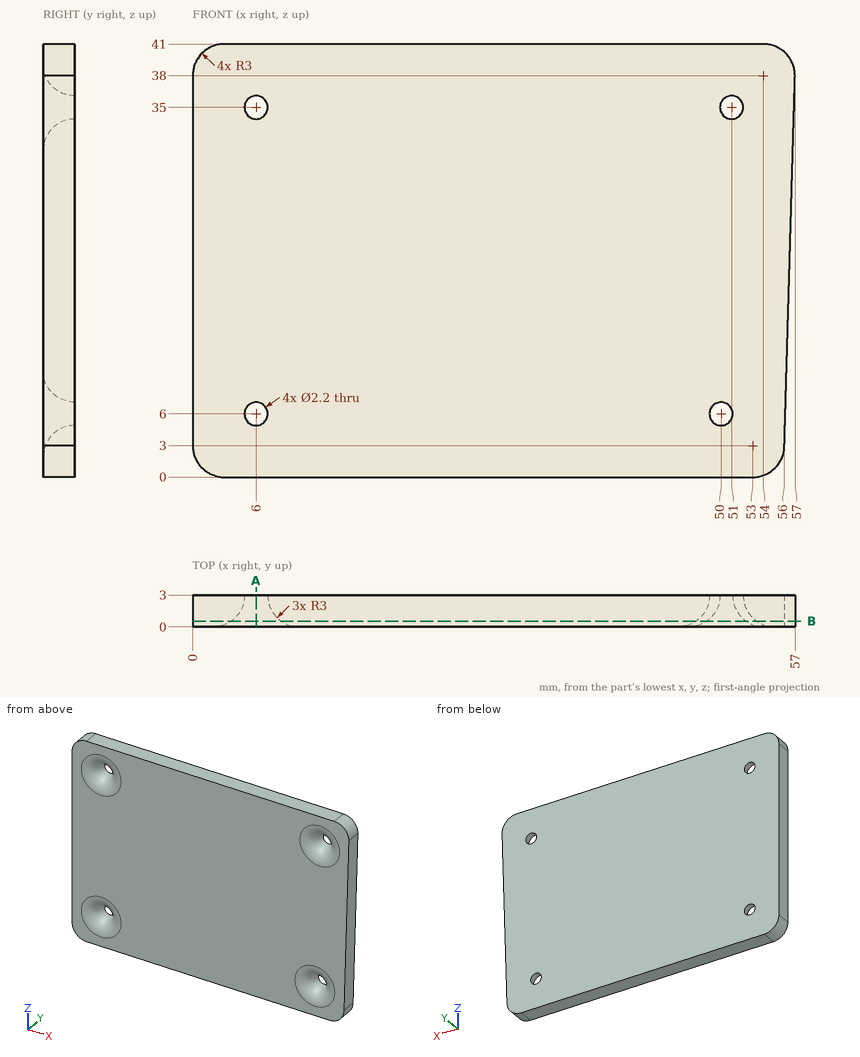
For this review, use the dimensioned drawing (mm, ordinates from the lowest corner) and the shaded views. Round coordinates to 2 decimals unless told otherwise and drop trailing zeros. Order: outer loops, then holes, each group sorted by start corner. A loop starts at its lowest first (then second) coordinate and runs counter-clockwise, first axis right, second up.
1) Consider section B-B (y = 0.55). State the section outline as (x, z) points.
The answers:
outline: (0, 3) arc R3 ccw to (3, 0) - (53, 0) arc R3 ccw to (56, 3) - (57, 38) arc R3 ccw to (54, 41) - (3, 41) arc R3 ccw to (0, 38) - close; hole circle Ø4.74 at (6, 6); hole circle Ø4.74 at (6, 35); hole circle Ø4.74 at (50, 6); hole circle Ø4.74 at (51, 35)
2) For L1, parallel to Z at x = 50, y = 2.05; L2, parallel to X at y = 0.5, z = 35; L3, parallel to Z at x = 51.5, y = 0.4, list the stretches that pass through material, from the lowest coordinate up.
The answers:
L1: z = 0 to 4.75, 7.25 to 34.24, 35.76 to 41
L2: x = 0 to 3.56, 8.44 to 48.56, 53.44 to 56.91
L3: z = 0 to 3.87, 8.13 to 32.45, 37.55 to 41
3) Clearance check with flat-ended pins moving along their axes: pin 1 Ø3 at (x, z) = (50, 6) entering from -Y; pin 2 Ø3.5 at (x, z) = (51, 35) entering from -Y; pin 3 Ø1.8 at (x, z) = (6, 35) entering from -Y; pin 4 Ø1 at (y, z) = (1.5, 28.5) entering from +X. State where each tip first meets the part, or that it passes through.
The answers:
pin 1: stops at y = 1.5
pin 2: stops at y = 1.14
pin 3: passes through
pin 4: stops at x = 56.74
4) Consider section A-A (x = 6). Count the separate pieces of the cut face and the enclosed holes in it, plus the area to 3 significant figures.
The answers:
separate pieces: 3
enclosed holes: 0
area: 102 mm2
